Read the model definition and answer for the solid it produces. Units are mm, in the model's axes. Face numbers are marked on the shaded views. A direction names the side the tool comes from. Give positions to 0.01 mm unless a question says otherwise; leave off trailing zeros. Loops run counter-clockwise (first coordinate to the right, second up) from the corner with the lowest first, then second, coordinate; pieces in that order, holes last. Notation, with made-up numbers: (39, 89) -> (71, 89) arc R24 cw to (71, 107) -> close; hole circle Ø10 at (-20, 7.5). An arc over 180 degrees is marked (long way). Return JSON: item names as keys, results as strings. Group by question number.
from build123d import *

# Parameters (mm, degrees)
F0_W     = 70
F0_H     = 20
F1_DEPTH = 4.7
F2_W     = 42
F2_H     = 20
F3_DEPTH = 3
F4_D     = 3.6
F4_DEPTH = 12
F5_D     = 4.6
F5_DEPTH = 12
F6_R     = 2


with BuildPart() as f1:
    # F0 (on Top) → F1 (new body)
    with BuildSketch(Plane.XY):
        Rectangle(F0_W, F0_H)
    extrude(amount=F1_DEPTH)

    # F2 (on face) → F3 (join)
    with BuildSketch(Plane.XY.offset(4.7)):
        Rectangle(F2_W, F2_H)
    extrude(amount=F3_DEPTH)

    # F4
    with Locations(Plane(origin=(0, 0, 0), x_dir=(1, 0, 0), z_dir=(0, 0, -1))):
        with Locations((-15.5, 0), (15.5, 0)):
            Hole(F4_D / 2, depth=F4_DEPTH)

    # F5
    with Locations(Plane(origin=(0, 0, 0), x_dir=(1, 0, 0), z_dir=(0, 0, -1))):
        with Locations((-30.5, 0), (30.5, 0)):
            Hole(F5_D / 2, depth=F5_DEPTH)

    # F6
    f6_edges = [f1.edges().sort_by_distance(p)[0] for p in [
        (35, -10, 2.35),
        (35, 10, 2.35),
        (-35, 10, 2.35),
        (-35, -10, 2.35),
    ]]
    fillet(f6_edges, radius=F6_R)


solid = f1.part
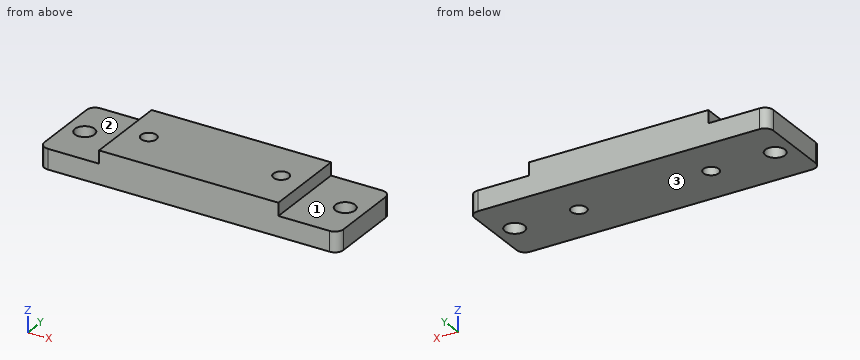
1. Section D-D on y = -4.75 is taken. Determine the outline of the cut face in (x, z), then the cut area to 3 significant figures.
2. Straight lines are drawn through the part: line 1 (Y direction, x = 30.5, z = 1.6); line 2 (X direction, y = 0.5, z = 3.25) (3 decimals); line 3 (Z direction, x = -28, y = 2.75). For each, find the intervals that lie inside material, in ascending order. Write a range as from..to.
3. Section C-C on x = 30.5 is taken. Determine the outline of the cut face in (y, z).
4. Section B-B on z = 3.75 is taken. Determine the outline of the cut face in (x, y).
5. Section A-A on y = 0 is taken. Determine the outline of the cut face in (x, z).
6. Flat-ended cylindrical pins translate along their axes: pin 1 Ø3 at (x, y) = (-15.5, 0) entering from +Z; pin 2 Ø5.5 at (x, y) = (-30.5, 0) entering from +Z; pin 3 Ø0.9 at (y, z) = (4.5, 6) entering from +X. Find the tip coordinate at first contact, or state that the pin passes through.
7. Which of the six approach directions +Z, -Z, +X, -X, +Y, -Y give full straight-line access (tool end or side, diameter ignored) to the marked faces 1, 2 and 3?
Completed:
{
 "1": {"outline": "(-35, 0) -> (35, 0) -> (35, 4.7) -> (21, 4.7) -> (21, 7.7) -> (-21, 7.7) -> (-21, 4.7) -> (-35, 4.7) -> close", "area": "455 mm²"},
 "2": {"line 1": "y = -10..-2.3, 2.3..10", "line 2": "x = -35..-32.745, -28.255..-17.229, -13.771..13.771, 17.229..28.255, 32.745..35", "line 3": "z = 0..4.7"},
 "3": {"outline": "(-10, 0) -> (-2.3, 0) -> (-2.3, 4.7) -> (-10, 4.7) -> close; (2.3, 0) -> (10, 0) -> (10, 4.7) -> (2.3, 4.7) -> close"},
 "4": {"outline": "(-35, -8) arc R2 ccw to (-33, -10) -> (33, -10) arc R2 ccw to (35, -8) -> (35, 8) arc R2 ccw to (33, 10) -> (-33, 10) arc R2 ccw to (-35, 8) -> close; hole circle Ø4.6 at (-30.5, 0); hole circle Ø3.6 at (-15.5, 0); hole circle Ø3.6 at (15.5, 0); hole circle Ø4.6 at (30.5, 0)"},
 "5": {"outline": "(-35, 0) -> (-32.8, 0) -> (-32.8, 4.7) -> (-35, 4.7) -> close; (-28.2, 0) -> (-17.3, 0) -> (-17.3, 7.7) -> (-21, 7.7) -> (-21, 4.7) -> (-28.2, 4.7) -> close; (-13.7, 0) -> (13.7, 0) -> (13.7, 7.7) -> (-13.7, 7.7) -> close; (17.3, 0) -> (28.2, 0) -> (28.2, 4.7) -> (21, 4.7) -> (21, 7.7) -> (17.3, 7.7) -> close; (32.8, 0) -> (35, 0) -> (35, 4.7) -> (32.8, 4.7) -> close"},
 "6": {"pin 1": "passes through", "pin 2": "stops at z = 4.7", "pin 3": "stops at x = 21"},
 "7": {"face 1": "+Z, +X, +Y, -Y", "face 2": "+Z, -X, +Y, -Y", "face 3": "-Z, +X, -X, +Y, -Y"}
}
